Read the model definition and answer for the solid it produces. Units are mm, in the model's axes. A direction names the side the tool comes from. Coordinates: 2 decimals unless noted, no trailing zeros. Write each loop counter-clockwise with the first axis right and the second up, starting at its lowest first coordinate (ties: lowest second). Pieces come first, ordered by that corner, then holes.
1) Find the intervals of material crossed by line 1 (Z direction, x = 1.15, y = 2); line 2 (Z direction, x = -0.3, y = -1.2); line 3 (Y direction, x = -0.05, z = -10.5), in increasing order.
2) The part is cut by section C-C (x = 0.3). Determine the outline of the cut face in (y, z), then the cut area to 3 significant figures.
3) Determine the mould class of faces 1 (the face through (0.6, 1.3, 3)), 2 (the face through (-0.596, -2.685, 1.479)), 3 (the face through (-0.63, -1.08, 2.26)), 4 (the face through (1.25, 0, 2)) for opening direction X: +X half, -X half, draft (parallel to the pull), parting line (faces both ways), or undercut.
4) The part is cut by section B-B (z = 2). Determine the outline of the cut face in (x, y), then the cut area to 3 significant figures.
5) Each of these flat-tipped pins is pushed along its axis until it touches: pin 1 Ø2 at (x, z) = (-2, -12) entering from +Y; pin 2 Ø2 at (x, z) = (-0.5, -4) entering from +Y; pin 3 Ø1.5 at (y, z) = (2, -8) entering from +X. Where does it stop, or does it pass through?
6) The part is cut by section D-D (z = -1.75). Determine the outline of the cut face in (x, y), then the cut area to 3 significant figures.
7) Which of the six approach directions +Z, -Z, +X, -X, +Y, -Y give full straight-line access (tool end or side, diameter ignored) to faces 5 (the face through (0.616, -1.088, 2.26)), 6 (the face through (1.5, 0.07, -6.9)), 7 (the face through (0, 0, -14))?
8) The part is cut by section A-A (y = 0). Determine the outline of the cut face in (x, z), then the cut area to 4 significant figures.
from build123d import *

# Parameters (mm, degrees)
SKETCH_1_R          = 2.75
EXTRUDE_1_DEPTH     = 3
CUT_EXTRUDE_1_DEPTH = 1.5
SKETCH_3_R          = 1.5
EXTRUDE_2_DEPTH     = 14


with BuildPart() as part:
    # 草图1 → 凸台-拉伸1 (new body)
    with BuildSketch(Plane.XY):
        Circle(SKETCH_1_R)
    extrude(amount=EXTRUDE_1_DEPTH)

    # 草图2 → 切除-拉伸1 (cut)
    with BuildSketch(Plane.XY.offset(3)):
        Polygon((0, -1.443375673), (1.25, -0.721687836), (1.25, 0.721687836), (0, 1.443375673), (-1.25, 0.721687836), (-1.25, -0.721687836), align=None)
    extrude(amount=-CUT_EXTRUDE_1_DEPTH, mode=Mode.SUBTRACT)

    # 草图3 → 凸台-拉伸2 (add)
    with BuildSketch(Plane(origin=(0, 0, 0), x_dir=(-1, 0, 0), z_dir=(0, 0, -1))):
        Circle(SKETCH_3_R)
    extrude(amount=EXTRUDE_2_DEPTH)


solid = part.part
Reported:
1. line 1: z = 0 to 3
1. line 2: z = -14 to 1.5
1. line 3: y = -1.5 to 1.5
2. outline: (-2.73, 0) - (-1.47, 0) - (-1.47, -14) - (1.47, -14) - (1.47, 0) - (2.73, 0) - (2.73, 3) - (1.27, 3) - (1.27, 1.5) - (-1.27, 1.5) - (-1.27, 3) - (-2.73, 3) - close
2. area: 53.7 mm2
3. face 1: draft
3. face 2: parting line
3. face 3: undercut
3. face 4: undercut
4. outline: circle Ø5.5 at (0, 0); hole (-1.25, -0.72) - (0, -1.44) - (1.25, -0.72) - (1.25, 0.72) - (0, 1.44) - (-1.25, 0.72) - close
4. area: 18.3 mm2
5. pin 1: stops at y = 1.12
5. pin 2: stops at y = 1.5
5. pin 3: stops at x = 0.83
6. outline: circle Ø3 at (0, 0)
6. area: 7.07 mm2
7. face 5: +Z
7. face 6: -Z
7. face 7: -Z, +X, -X, +Y, -Y
8. outline: (-2.75, 0) - (-1.5, 0) - (-1.5, -14) - (1.5, -14) - (1.5, 0) - (2.75, 0) - (2.75, 3) - (1.25, 3) - (1.25, 1.5) - (-1.25, 1.5) - (-1.25, 3) - (-2.75, 3) - close
8. area: 54.75 mm2
